Design review of the part built by this model. Coordinates are the model's own, in mm. A direction names the side the tool comes from. Give positions to 0.01 mm unless a question says otherwise; leave off trailing zeros. Order: outer loops, then holes, each group sorted by start corner. A loop starts at its lowest first (then second) coordinate and runs counter-clockwise, first axis right, second up. Notation, with made-up numbers: (73.25, 49.5) -> (79.25, 49.5) arc R28 cw to (79.25, 67.5) -> close; hole circle Ø6 at (12, 83). An arc over 180 degrees is marked (long way). Return JSON: item names as keys, results as strings.
```python
from build123d import *

# Parameters (mm, degrees)
SKETCH1_R           = 1.5
BOSS_EXTRUDE1_DEPTH = 2
SKETCH2_W           = 6
SKETCH2_H           = 12
BOSS_EXTRUDE2_DEPTH = 12
SKETCH3_W           = 2
SKETCH3_H           = 4
BOSS_EXTRUDE3_DEPTH = 2


with BuildPart() as part:
    # Sketch1 → Boss-Extrude1 (new body)
    with BuildSketch(Plane(origin=(0, 0, 0), x_dir=(1, 0, 0), z_dir=(0, 1, 0))):
        with BuildLine():
            Line((-7, 11), (7, 11))
            ThreePointArc((7, 11), (9.121320344, 10.121320344), (10, 8))
            Line((10, 8), (10, -8))
            ThreePointArc((10, -8), (9.121320344, -10.121320344), (7, -11))
            Line((7, -11), (-7, -11))
            ThreePointArc((-7, -11), (-9.121320344, -10.121320344), (-10, -8))
            Line((-10, -8), (-10, 8))
            ThreePointArc((-10, 8), (-9.121320344, 10.121320344), (-7, 11))
        make_face()
        with Locations(Location((7, 8, 0), (0, 0, 270))):
            Circle(SKETCH1_R, mode=Mode.SUBTRACT)
        with Locations(Location((7, -8, 0), (0, 0, 270))):
            Circle(SKETCH1_R, mode=Mode.SUBTRACT)
    extrude(amount=BOSS_EXTRUDE1_DEPTH)

    # Sketch2 → Boss-Extrude2 (add)
    with BuildSketch(Plane(origin=(0, 2, 0), x_dir=(1, 0, 0), z_dir=(0, 1, 0))):
        with Locations((-7, 0)):
            Rectangle(SKETCH2_W, SKETCH2_H)
    extrude(amount=BOSS_EXTRUDE2_DEPTH)

    # Sketch3 → Boss-Extrude3 (add)
    with BuildSketch(Plane.XZ):
        with Locations((2, 0)):
            Rectangle(SKETCH3_W, SKETCH3_H)
    extrude(amount=BOSS_EXTRUDE3_DEPTH)


solid = part.part
```
Item 1: Add section C-C (y = 7.5). Give the boundary of the cut face in (x, z).
Result set:
{"outline": "(-10, -6) -> (-4, -6) -> (-4, 6) -> (-10, 6) -> close"}
Item 2: Add section B-B (z = -1.5). Give the boundary of the cut face in (x, y).
Result set:
{"outline": "(-10, 0) -> (1, 0) -> (1, -2) -> (3, -2) -> (3, 0) -> (10, 0) -> (10, 2) -> (-4, 2) -> (-4, 14) -> (-10, 14) -> close"}
Item 3: Wall thickness on L1, parallel to X at y = 1.1, z = -8; L2, parallel to Y at x = 8.75, z = -1; L3, parallel to Z at x = 6.75, y = 0.5: over which ranges is each line inside the solid? List them lowest first. Write a range as [from, to].
Result set:
{"L1": "x = [-10, 5.5], [8.5, 10]", "L2": "y = [0, 2]", "L3": "z = [-11, -9.48], [-6.52, 6.52], [9.48, 11]"}
Item 4: Add section A-A (x = -6). Give the boundary of the cut face in (y, z).
Result set:
{"outline": "(0, -11) -> (2, -11) -> (2, -6) -> (14, -6) -> (14, 6) -> (2, 6) -> (2, 11) -> (0, 11) -> close"}
Item 5: For pin 1 (2 mm diameter, centred on y = 7, z = -5.5, fed in from +X); pin 2 (2 mm diameter, centred on y = -0.5, z = 0.5, fed in from -X); pin 3 (3.5 mm diameter, centred on x = 7, z = 8, fed in from -Y); pin 4 (1 mm diameter, centred on x = 1.5, y = -1, fed in from -Z), all flat-tipped, find the tip position at first contact; note any pin that passes through.
Result set:
{"pin 1": "stops at x = -4", "pin 2": "stops at x = -10", "pin 3": "stops at y = 0", "pin 4": "stops at z = -2"}
Item 6: Add section D-D (z = -4.5). Give the boundary of the cut face in (x, y), plus the area to 3 significant figures.
Result set:
{"outline": "(-10, 0) -> (10, 0) -> (10, 2) -> (-4, 2) -> (-4, 14) -> (-10, 14) -> close", "area": "112 mm^2"}
Item 7: Machinability: for faces 1 (the face through (2, -1, 2)), 2 (the face through (3, -1, 0)), 3 (the face through (2, -1, -2)), 4 (the face through (-7, 8, 6)), 5 (the face through (-4, 8, 0)), which of the approach directions +Z, -Z, +X, -X, +Y, -Y give a long, thin tool a straight path to every point of the face, cutting with its end or side? Answer none if there is none.
Result set:
{"face 1": "+Z, +X, -X, -Y", "face 2": "+Z, -Z, +X, -Y", "face 3": "-Z, +X, -X, -Y", "face 4": "+Z, +X, -X, +Y", "face 5": "+Z, -Z, +X, +Y"}
